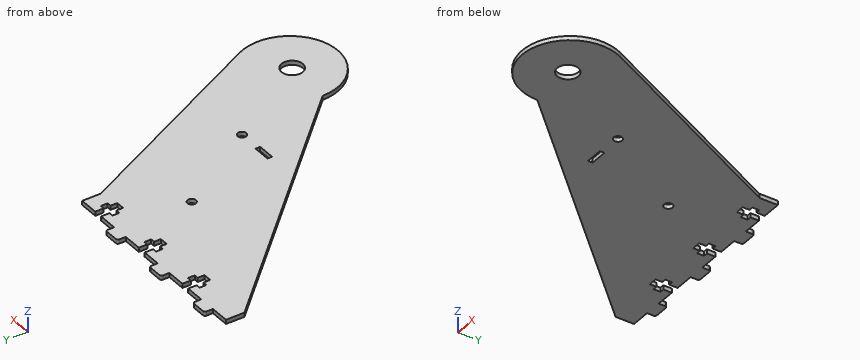
from build123d import *

# Parameters (mm, degrees)
SKETCH_1_R      = 2
SKETCH_1_R_2    = 5.02
SKETCH_1_W      = 8.2
SKETCH_1_H      = 2.2
EXTRUDE_1_DEPTH = 2
FILLET_1_R      = 1


with BuildPart() as part:
    # 草图1 → 凸台-拉伸1 (new body)
    with BuildSketch(Plane.XY):
        with BuildLine():
            Line((-38.15, 66.25), (-38.15, 62.25))
            Line((-38.15, 62.25), (-40.15, 62.25))
            Line((-40.15, 62.25), (-40.15, 59.05))
            Line((-40.15, 59.05), (-38.15, 59.05))
            Line((-38.15, 59.05), (-38.15, 55.85))
            Line((-38.15, 55.85), (-34.15, 55.85))
            Line((-34.15, 55.85), (-34.15, 59.05))
            Line((-34.15, 59.05), (-32.15, 59.05))
            Line((-32.15, 59.05), (-32.15, 62.25))
            Line((-32.15, 62.25), (-34.15, 62.25))
            Line((-34.15, 62.25), (-34.15, 66.25))
            Line((-34.15, 66.25), (-25.15, 66.25))
            Line((-25.15, 66.25), (-25.15, 70.25))
            Line((-25.15, 70.25), (-17.15, 70.25))
            Line((-17.15, 70.25), (-17.15, 66.25))
            Line((-17.15, 66.25), (-8.15, 66.25))
            Line((-8.15, 66.25), (-8.15, 62.25))
            Line((-8.15, 62.25), (-10.15, 62.25))
            Line((-10.15, 62.25), (-10.15, 59.05))
            Line((-10.15, 59.05), (-8.15, 59.05))
            Line((-8.15, 59.05), (-8.15, 55.85))
            Line((-8.15, 55.85), (-4.15, 55.85))
            Line((-4.15, 55.85), (-4.15, 59.05))
            Line((-4.15, 59.05), (-2.15, 59.05))
            Line((-2.15, 59.05), (-2.15, 62.25))
            Line((-2.15, 62.25), (-4.15, 62.25))
            Line((-4.15, 62.25), (-4.15, 66.25))
            Line((-4.15, 66.25), (4.85, 66.25))
            Line((4.85, 66.25), (4.85, 57.55))
            Line((4.85, 57.55), (54.01460577, -41.768082641))
            ThreePointArc((54.01460577, -41.768082641), (38.975737517, -73.658373169), (11.35, -51.75))
            Line((11.35, -51.75), (-94.15, 57.55))
            Line((-94.15, 57.55), (-94.15, 66.25))
            Line((-94.15, 66.25), (-85.15, 66.25))
            Line((-85.15, 66.25), (-85.15, 70.25))
            Line((-85.15, 70.25), (-77.15, 70.25))
            Line((-77.15, 70.25), (-77.15, 66.25))
            Line((-77.15, 66.25), (-68.15, 66.25))
            Line((-68.15, 66.25), (-68.15, 62.25))
            Line((-68.15, 62.25), (-70.15, 62.25))
            Line((-70.15, 62.25), (-70.15, 59.05))
            Line((-70.15, 59.05), (-68.15, 59.05))
            Line((-68.15, 59.05), (-68.15, 55.85))
            Line((-68.15, 55.85), (-64.15, 55.85))
            Line((-64.15, 55.85), (-64.15, 59.05))
            Line((-64.15, 59.05), (-62.15, 59.05))
            Line((-62.15, 59.05), (-62.15, 62.25))
            Line((-62.15, 62.25), (-64.15, 62.25))
            Line((-64.15, 62.25), (-64.15, 66.25))
            Line((-64.15, 66.25), (-55.15, 66.25))
            Line((-55.15, 66.25), (-55.15, 70.25))
            Line((-55.15, 70.25), (-47.15, 70.25))
            Line((-47.15, 70.25), (-47.15, 66.25))
            Line((-47.15, 66.25), (-38.15, 66.25))
        make_face()
        with Locations((-19.762745434, 31.422010331)):
            Circle(SKETCH_1_R, mode=Mode.SUBTRACT)
        with Locations((7.098407643, -10.75)):
            Circle(SKETCH_1_R, mode=Mode.SUBTRACT)
        with Locations((33.85, -52.75)):
            Circle(SKETCH_1_R_2, mode=Mode.SUBTRACT)
        with Locations((-7.901592357, -10.75)):
            Rectangle(SKETCH_1_W, SKETCH_1_H, mode=Mode.SUBTRACT)
    extrude(amount=EXTRUDE_1_DEPTH)

    # 圆角1
    fillet_1_edges = [part.edges().sort_by_distance(p)[0] for p in [
        (-25.15, 70.25, 1),
        (-17.15, 70.25, 1),
        (-85.15, 70.25, 1),
        (-77.15, 70.25, 1),
        (-55.15, 70.25, 1),
        (-47.15, 70.25, 1),
    ]]
    fillet(fillet_1_edges, radius=FILLET_1_R)


solid = part.part
Source: CAD feature listing. Evaluate the final solid. Frame: model axes, mm. Give positions to 0.01 mm unless a question says otherwise; leave off trailing zeros. Write each loop counter-clockwise with the first axis right and the second up, starting at its lowest first coordinate (ties: lowest second). Pieces come first, ordered by that corner, then holes. Notation, with made-up numbers: M 37,36 L 47,36 A31 cw 47,64 Z; hole C 69,39.25 d5. An arc over 180 degrees is marked long. Return JSON: item names as keys, results as strings. Group by question number.
1) Cut plane B-B, the plane z = 0.4. Give the number of separate pieces and of enclosed holes in the cut face, plus the area to 3 significant figures.
2) Pin query (flat end, axial travel): P1, Ø1, axis at x = -62.5, z = 0.5, coming from the -Y side; P2, Ø0.6, axis at y = 61.5, z = 1, coming from the +X side; P3, Ø5, axis at x = 7.1, y = -10.75, coming from the -Z side; P4, Ø0.6, axis at x = -3, z = 1.5, coming from the +Y side. Return the tip coordinate at first contact, or that it passes through.
3) Cut plane A-A, the plane x = 33.85. Output: boundary loops of the cut face in (y, z).
4) Cut plane C-C, the plane y = 19. Output: boundary loops of the cut face in (x, z).
5) Material intervals for line 1 along X through (y, z) = (57, 0.5); line 2 along X through (y, z) = (57.5, 0.2); line 3 along X through (y, z) = (-57, 0.25), sorted ascending. Write a range as [from, to].
6) Cut plane D-D, the plane x = 3. Output: boundary loops of the cut face in (y, z), plus the area to 3 significant figures.
Recorded:
{
 "1": {"separate pieces": "1", "enclosed holes": "4", "area": "9,470 mm²"},
 "2": {"P1": "stops at y = 24.24", "P2": "stops at x = 4.85", "P3": "stops at z = 0", "P4": "stops at y = 66.25"},
 "3": {"outline": "M -74.25,0 L -57.77,0 L -57.77,2 L -74.25,2 Z; M -47.73,0 L -1.03,0 L -1.03,2 L -47.73,2 Z"},
 "4": {"outline": "M -56.94,0 L 23.93,0 L 23.93,2 L -56.94,2 Z"},
 "5": {"line 1": "x = [-93.62, -68.15], [-64.15, -38.15], [-34.15, -8.15], [-4.15, 5.12]", "line 2": "x = [-94.1, -68.15], [-64.15, -38.15], [-34.15, -8.15], [-4.15, 4.87]", "line 3": "x = [11.97, 31.18], [36.52, 55.73]"},
 "6": {"outline": "M -43.1,0 L 66.25,0 L 66.25,2 L -43.1,2 Z", "area": "219 mm²"}
}
